Design review of the part built by this model. Coordinates are the model's own, in mm. Face numbers are marked on the shaded views. Give positions to 0.01 mm unless a question says otherwise; leave off trailing zeros. Write each loop counter-clockwise with the first axis right and the second up, starting at its lowest first coordinate (ties: lowest second). Pieces come first, ordered by that corner, then holes. Notation, with made-up numbers: (4.5, -6.5) -> (42.5, -6.5) arc R11 ccw to (42.5, 2.5) -> close; hole circle Ø7 at (5, 59.5). An arc over 180 degrees is marked (long way). Use CSV: the item, a comma, the result in double quotes.
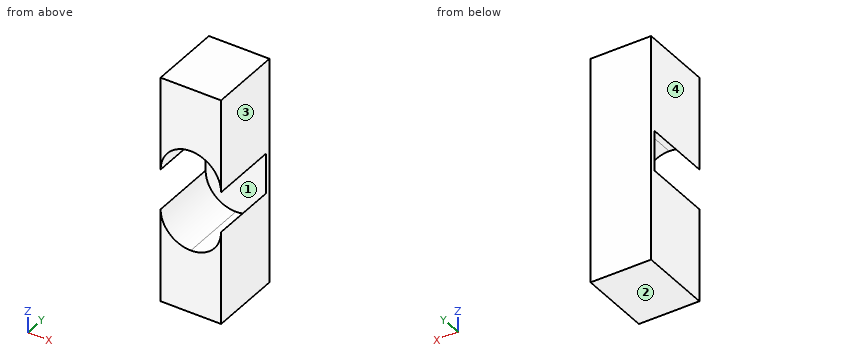
```python
from build123d import *

# Parameters (mm, degrees)
F0_W     = 12
F0_H     = 45
F1_DEPTH = 14.5
F3_DEPTH = 13.5


with BuildPart() as f1:
    # F0 (on Front) → F1 (new body)
    with BuildSketch(Plane.XZ):
        with Locations((-33.3756405115, 57.3880812526)):
            Rectangle(F0_W, F0_H)
    extrude(amount=F1_DEPTH)

    # F2 (on face) → F3 (cut)
    with BuildSketch(Plane.XZ.offset(14.5)):
        with BuildLine():
            ThreePointArc((-37.8477764665, 57.3880812526), (-38.9806746653, 59.2471487139), (-39.3756405115, 61.3880812526))
            Line((-39.3756405115, 61.3880812526), (-39.3756405115, 53.3880812526))
            ThreePointArc((-39.3756405115, 53.3880812526), (-38.9806746653, 55.5290137912), (-37.8477764665, 57.3880812526))
        make_face()
        with BuildLine():
            Line((-27.3756405115, 53.3880812526), (-27.3756405115, 61.3880812526))
            ThreePointArc((-27.3756405115, 61.3880812526), (-27.7706063577, 59.2471487139), (-28.9035045565, 57.3880812526))
            ThreePointArc((-28.9035045565, 57.3880812526), (-27.7706063577, 55.5290137912), (-27.3756405115, 53.3880812526))
        make_face()
        with BuildLine():
            ThreePointArc((-27.3756405115, 61.3880812526), (-29.1329998244, 65.6307219397), (-33.3756405115, 67.3880812526))
            ThreePointArc((-33.3756405115, 67.3880812526), (-37.6182811986, 65.6307219397), (-39.3756405115, 61.3880812526))
            ThreePointArc((-39.3756405115, 61.3880812526), (-38.9806746653, 59.2471487139), (-37.8477764665, 57.3880812526))
            ThreePointArc((-37.8477764665, 57.3880812526), (-33.3756405115, 59.3880812526), (-28.9035045565, 57.3880812526))
            ThreePointArc((-28.9035045565, 57.3880812526), (-27.7706063577, 59.2471487139), (-27.3756405115, 61.3880812526))
        make_face()
        with BuildLine():
            ThreePointArc((-37.8477764665, 57.3880812526), (-38.9806746653, 55.5290137912), (-39.3756405115, 53.3880812526))
            ThreePointArc((-39.3756405115, 53.3880812526), (-37.6182811986, 49.1454405655), (-33.3756405115, 47.3880812526))
            ThreePointArc((-33.3756405115, 47.3880812526), (-29.1329998244, 49.1454405655), (-27.3756405115, 53.3880812526))
            ThreePointArc((-27.3756405115, 53.3880812526), (-27.7706063577, 55.5290137912), (-28.9035045565, 57.3880812526))
            ThreePointArc((-28.9035045565, 57.3880812526), (-33.3756405115, 55.3880812526), (-37.8477764665, 57.3880812526))
        make_face()
        with BuildLine():
            ThreePointArc((-28.9035045565, 57.3880812526), (-33.3756405115, 59.3880812526), (-37.8477764665, 57.3880812526))
            ThreePointArc((-37.8477764665, 57.3880812526), (-33.3756405115, 55.3880812526), (-28.9035045565, 57.3880812526))
        make_face()
    extrude(amount=-F3_DEPTH, mode=Mode.SUBTRACT)


solid = f1.part
```
(1) Take a section at C-C (z = 48). Write out the cut boundary in (x, y), then the cut area to 3 significant figures.
Established:
outline,"(-39.38, -14.5) -> (-36.02, -14.5) -> (-36.02, -1) -> (-30.74, -1) -> (-30.74, -14.5) -> (-27.38, -14.5) -> (-27.38, 0) -> (-39.38, 0) -> close"
area,"103 mm2"
(2) Clearance check with a flat-ended pin moving along its axis: pin 1 (1 mm diameter, centred on x = -30, z = 61, fed in from -Y). State where the tip first meets the part, or that it passes through.
Established:
pin 1,"stops at y = -1"
(3) For line 1 along Y through (x, z) = (-32.75, 60); line 2 along Z through (x, y) = (-38.5, -5.25); line 3 along Z through (x, y) = (-32.25, -7.5), list the stretches that pass through material, from the lowest coordinate up. Write a range as [from, to].
Established:
line 1,"y = [-1, 0]"
line 2,"z = [34.89, 50.27], [64.51, 79.89]"
line 3,"z = [34.89, 47.49], [67.28, 79.89]"
(4) Take a section at A-A (y = -8). Write out the cut boundary in (x, z).
Established:
outline,"(-39.38, 34.89) -> (-27.38, 34.89) -> (-27.38, 53.39) arc R6 cw to (-39.38, 53.39) -> close; (-39.38, 61.39) arc R6 cw to (-27.38, 61.39) -> (-27.38, 79.89) -> (-39.38, 79.89) -> close"
(5) Take a section at B-B (x = -30.25). Write out the cut boundary in (y, z).
Established:
outline,"(-14.5, 34.89) -> (0, 34.89) -> (0, 79.89) -> (-14.5, 79.89) -> (-14.5, 66.51) -> (-1, 66.51) -> (-1, 48.27) -> (-14.5, 48.27) -> close"
(6) Mouldability with a two-part tool opening along X and no side actions: class the marked faces 1, 2, 3 and 4 as +X half, -X half, draft (parallel to the pull), parting line (faces both ways), or undercut.
Established:
face 1,"undercut"
face 2,"draft"
face 3,"+X half"
face 4,"-X half"
